Solid Edge part; units mm, degrees
sketch "Sketch1" plane through (0, 0, 0) normal (0, 0, -1) x (-1, 0, 0)
  line L0 (-3.9, -3.85) -> (3.9, -3.85)
  line L1 (3.9, -3.85) -> (3.9, 3.85)
  line L2 (3.9, 3.85) -> (-3.9, 3.85)
  line L3 (-3.9, 3.85) -> (-3.9, -3.85)
extrude "Protrusion1" add sketch "Sketch1" against normal blind 5.97
sketch "Sketch2" plane through (0, -3.85, 2.985) normal (0, -1, 0) x (1, 0, 0)
  line L0 (-3.9, 2.985) -> (3.9, 2.985)
  line L1 (3.9, 2.985) -> (3.9, -1.045)
  line L2 (3.9, -1.045) -> (-3.9, 2.985)
extrude "ExtrudedCutout_1" cut sketch "Sketch2" against normal blind 12.0859
sketch "Sketch3" plane through (0, -3.85, 2.985) normal (0, -1, 0) x (1, 0, 0)
  line L0 (3.9, -2.585) -> (3.9, -3.3266)
  line L1 (3.9, -3.3266) -> (-3.9, -3.3266)
  line L2 (-3.9, -2.585) -> (-3.9, -3.3266)
  line L3 (-3.9, -2.585) -> (-3.6, -2.585)
  line L4 (-3.6, -2.585) -> (-3.6, -2.985)
  line L5 (3.6, -2.985) -> (-3.6, -2.985)
  line L6 (3.6, -2.585) -> (3.6, -2.985)
  line L7 (3.9, -2.585) -> (3.6, -2.585)
extrude "ExtrudedCutout_2" cut sketch "Sketch3" against normal blind 9.1473
sketch "Sketch4" plane through (0, 0, 0) normal (0, 0, -1) x (0, -1, 0)
  line L0 (-2.4, -2.4) -> (2.4, -2.4)
  line L1 (2.4, -2.4) -> (2.4, 2.4)
  line L2 (2.4, 2.4) -> (-2.4, 2.4)
  line L3 (-2.4, 2.4) -> (-2.4, -2.4)
extrude "ExtrudedCutout_4" cut sketch "Sketch4" against normal blind 1.8
sketch "Sketch5" plane through (-3.9, 0, 3.185) normal (-1, 0, 0) x (0, -1, 0)
  line L0 (3.85, -2.785) -> (3.6, -2.785)
  line L1 (3.6, -2.785) -> (3.6, -3.185)
  line L2 (-3.6, -3.185) -> (3.6, -3.185)
  line L3 (-3.6, -2.785) -> (-3.6, -3.185)
  line L4 (-3.85, -2.785) -> (-3.6, -2.785)
  line L5 (-3.85, -3.5485) -> (-3.85, -2.785)
  line L6 (3.85, -3.5485) -> (-3.85, -3.5485)
  line L7 (3.85, -2.785) -> (3.85, -3.5485)
extrude "ExtrudedCutout_5" cut sketch "Sketch5" against normal blind 8.7278
For this review, take the finished solid that the model builds, in its own axes (mm). A direction names the side the tool comes from. Coordinates: 2 decimals unless noted, no trailing zeros. Write each loop counter-clockwise with the first axis right and the second up, starting at its lowest first coordinate (ties: lowest second). Pieces come first, ordered by that corner, then holes.
(1) Add section B-B on x = 1.5. Give the boundary of the cut face in (y, z), then the cut area to 3 significant figures.
(2) Wall thickness on probe 1 along X at (y, z) = (2.25, 1.4); probe 2 along Y at (x, z) = (0.25, 1.2); probe 3 along Z at (x, y) = (2.5, -2.5): over which ranges is each line inside the solid? List them lowest first.
(3) Add section A-A on z = 0.8. Give the boundary of the cut face in (x, y), then the cut area to 3 significant figures.
(4) Tool access review of faces 4 (the face through (2.4, 0, 1)), 5 (the face through (3.9, 0, 1)): name each direction out of +Z, -Z, +X, -X, +Y, -Y from which nothing blocks a thin tool from reaching the whole face with its end or side.
(5) Add section D-D on x = -3. Give the boundary of the cut face in (y, z) (3 decimals), then the cut area to 3 significant figures.
(6) For pin 1 Ø2 at (y, z) = (2, 3) entering from +X, flat-tipped, find the tip position at first contact; note if it passes through.
(7) The part is to be moulded in two halves that separate along X. For faces 1 (the face through (0, 0, 1.8)), 2 (the face through (-3.9, 0, 3)), 3 (the face through (-1, 3.85, 3)), say which applies: +X half, -X half, draft (parallel to the pull), parting line (faces both ways), or undercut.
(8) Add section C-C on y = 2.25. Give the boundary of the cut face in (x, z), then the cut area to 3 significant figures.
Answer sheet:
1. outline: (-3.85, 0.4) - (-3.6, 0.4) - (-3.6, 0) - (-2.4, 0) - (-2.4, 1.8) - (2.4, 1.8) - (2.4, 0) - (3.6, 0) - (3.6, 0.4) - (3.85, 0.4) - (3.85, 3.18) - (-3.85, 3.18) - close
1. area: 15.6 mm2
2. probe 1: x = -3.9 to -2.4, 2.4 to 3.9
2. probe 2: y = -3.85 to -2.4, 2.4 to 3.85
2. probe 3: z = 0 to 2.66
3. outline: (-3.9, -3.85) - (3.9, -3.85) - (3.9, 3.85) - (-3.9, 3.85) - close; hole (-2.4, -2.4) - (2.4, -2.4) - (2.4, 2.4) - (-2.4, 2.4) - close
3. area: 37.0 mm2
4. face 4: -Z
4. face 5: +Z, -Z, +X, +Y, -Y
5. outline: (-3.85, 0.4) - (-3.6, 0.4) - (-3.6, 0) - (3.6, 0) - (3.6, 0.4) - (3.85, 0.4) - (3.85, 5.505) - (-3.85, 5.505) - close
5. area: 42.2 mm2
6. pin 1: stops at x = 3.78
7. face 1: undercut
7. face 2: -X half
7. face 3: draft
8. outline: (-3.9, 0.4) - (-3.6, 0.4) - (-3.6, 0) - (-2.4, 0) - (-2.4, 1.8) - (2.4, 1.8) - (2.4, 0) - (3.6, 0) - (3.6, 0.4) - (3.9, 0.4) - (3.9, 1.94) - (-3.9, 5.97) - close
8. area: 22.0 mm2
